```python
from build123d import *

# Parameters (mm, degrees)
F1_DEPTH = 9.525
F2_W     = 203.2
F2_H     = 9.525
F3_DEPTH = 9.525
F4_W     = 19.05
F4_H     = 76.2
F5_DEPTH = 88.9
F7_DEPTH = 123.826


with BuildPart() as f1:
    # F0 (on Front) → F1 (new body)
    with BuildSketch(Plane.XZ):
        with BuildLine():
            Line((140.682878, 9.299915), (-62.517122, 9.299915))
            Line((-62.517122, 9.299915), (-62.517122, -41.500085))
            ThreePointArc((-62.517122, -41.500085), (-44.55661, -48.939573), (-37.117122, -66.900085))
            Line((-37.117122, -66.900085), (13.682878, -66.900085))
            ThreePointArc((13.682878, -66.900085), (39.082878, -92.300085), (64.482878, -66.900085))
            Line((64.482878, -66.900085), (115.282878, -66.900085))
            ThreePointArc((115.282878, -66.900085), (122.722366, -48.939573), (140.682878, -41.500085))
            Line((140.682878, -41.500085), (140.682878, 9.299915))
        make_face()
    extrude(amount=F1_DEPTH)

    # F2 (on face) → F3 (join)
    with BuildSketch(Plane.XY.offset(9.299915)):
        with Locations((39.082878, -4.7625)):
            Rectangle(F2_W, F2_H)
        with BuildLine():
            Line((-75.217122, -9.525), (-62.517122, -9.525))
            Line((-62.517122, -9.525), (-62.517122, 0))
            Line((-62.517122, 0), (140.682878, 0))
            Line((140.682878, 0), (140.682878, -9.525))
            Line((140.682878, -9.525), (153.382878, -9.525))
            Line((153.382878, -9.525), (153.382878, 79.784349))
            ThreePointArc((153.382878, 79.784349), (145.94339, 97.744861), (127.982878, 105.184349))
            Line((127.982878, 105.184349), (-49.817122, 105.184349))
            ThreePointArc((-49.817122, 105.184349), (-67.777634, 97.744861), (-75.217122, 79.784349))
            Line((-75.217122, 79.784349), (-75.217122, -9.525))
        make_face()
    extrude(amount=F3_DEPTH)

    # F4 (on face) → F5 (join)
    with BuildSketch(Plane(origin=(0, 0, 0), x_dir=(-1, 0, 0), z_dir=(0, 1, 0))):
        with Locations((-39.082878, -28.800085)):
            Rectangle(F4_W, F4_H)
    extrude(amount=F5_DEPTH)

    # F6 (on face) → F7 (cut, through all)
    with BuildSketch(Plane.YZ.offset(48.607878)):
        with BuildLine():
            ThreePointArc((19.05, -66.900085), (82.336633, -128.35491), (144.408027, -65.672893))
            ThreePointArc((144.408027, -65.672893), (128.516712, -23.962451), (88.9, -3.400085))
            ThreePointArc((88.9, -3.400085), (39.556499, -19.289734), (19.05, -66.900085))
        make_face()
    extrude(amount=-F7_DEPTH, mode=Mode.SUBTRACT)


solid = f1.part
```
Model file for the job. Use its own axes, mm. A direction names the side the tool comes from. Coordinates: 2 decimals unless noted, no trailing zeros. Loops run counter-clockwise (first coordinate to the right, second up) from the corner with the lowest first, then second, coordinate; pieces in that order, holes last. Notation, with made-up numbers: (41.25, -2.5) - (46.25, -2.5) arc R34 ccw to (46.25, 36.5) - close; hole circle Ø6 at (-4.5, -17.75). An arc over 180 degrees is marked (long way). Answer as a JSON object with one key per item and string values. Group by question number.
(1) Cut at C-C (y = 23.5). Give the cut face in (x, z).
(2) Probe line 1 along Z through (x, y) = (81, 61.5); line 2 along Y through (x, z) = (110, -25) (3 decimals); line 3 along X through (y, z) = (12.5, -36.5). List the from-to ranges inside material, lowest first.
(3) Cut at A-A (x = -8). Give the cut face in (y, z) (3 decimals).
(4) Cut at B-B (z = -22.5). Give the cut face in (x, y) (3 decimals), then the cut area to 3 significant figures.
(5) Tool access for faces 1 (the face through (39, 9, -66.9)), 2 (the face through (140.683, -5, -16)), 3 (the face through (-12, -5, -66.9)): list every direction of +Z, -Z, +X, -X, +Y, -Y with a clear straight run to the whole face (end or side of a thin tool).
(6) Flat gauge pins, fed straight in: pin 1 (6.5 mm diameter, centred on x = 37.5, z = 2.5, fed in from +Y); pin 2 (3 mm diameter, centred on x = 92, y = -5, fed in from -Z); pin 3 (10.5 mm diameter, centred on y = -2.5, z = -15.5, fed in from +X). Where does each tip first touch, or does it go through?
(7) Cut at D-D (x = 53.5). Give the cut face in (y, z) (3 decimals), then the cut area to 3 significant figures.
Geometry says:
{
 "1": {"outline": "(-75.22, 9.3) - (29.56, 9.3) - (29.56, -42.45) - (48.61, -42.45) - (48.61, 9.3) - (153.38, 9.3) - (153.38, 18.82) - (-75.22, 18.82) - close"},
 "2": {"line 1": "z = 9.3 to 18.82", "line 2": "y = -9.525 to 0", "line 3": "x = 29.56 to 48.61"},
 "3": {"outline": "(-9.525, -66.9) - (0, -66.9) - (0, 9.3) - (105.184, 9.3) - (105.184, 18.825) - (-9.525, 18.825) - close"},
 "4": {"outline": "(-62.517, -9.525) - (140.683, -9.525) - (140.683, 0) - (48.608, 0) - (48.608, 36.275) - (29.558, 36.275) - (29.558, 0) - (-62.517, 0) - close", "area": "2,630 mm^2"},
 "5": {"face 1": "-Z, +X, -X, +Y", "face 2": "-Z, +X, +Y, -Y", "face 3": "-Z, -X, +Y, -Y"},
 "6": {"pin 1": "stops at y = 88.9", "pin 2": "stops at z = -66.9", "pin 3": "stops at x = 140.68"},
 "7": {"outline": "(-9.525, -87.812) - (0, -87.812) - (0, 9.3) - (105.184, 9.3) - (105.184, 18.825) - (-9.525, 18.825) - close", "area": "2,020 mm^2"}
}
